For this review, use the dimensioned drawing (mm, ordinates from the lowest corner) and the shaded views. Round coordinates to 2 decimals unless told otherwise and drop trailing zeros. Write each loop counter-clockwise with the first axis right and the second up, starting at its lowest first coordinate (ties: lowest second). Pieces come first, ordered by that corner, then holes.
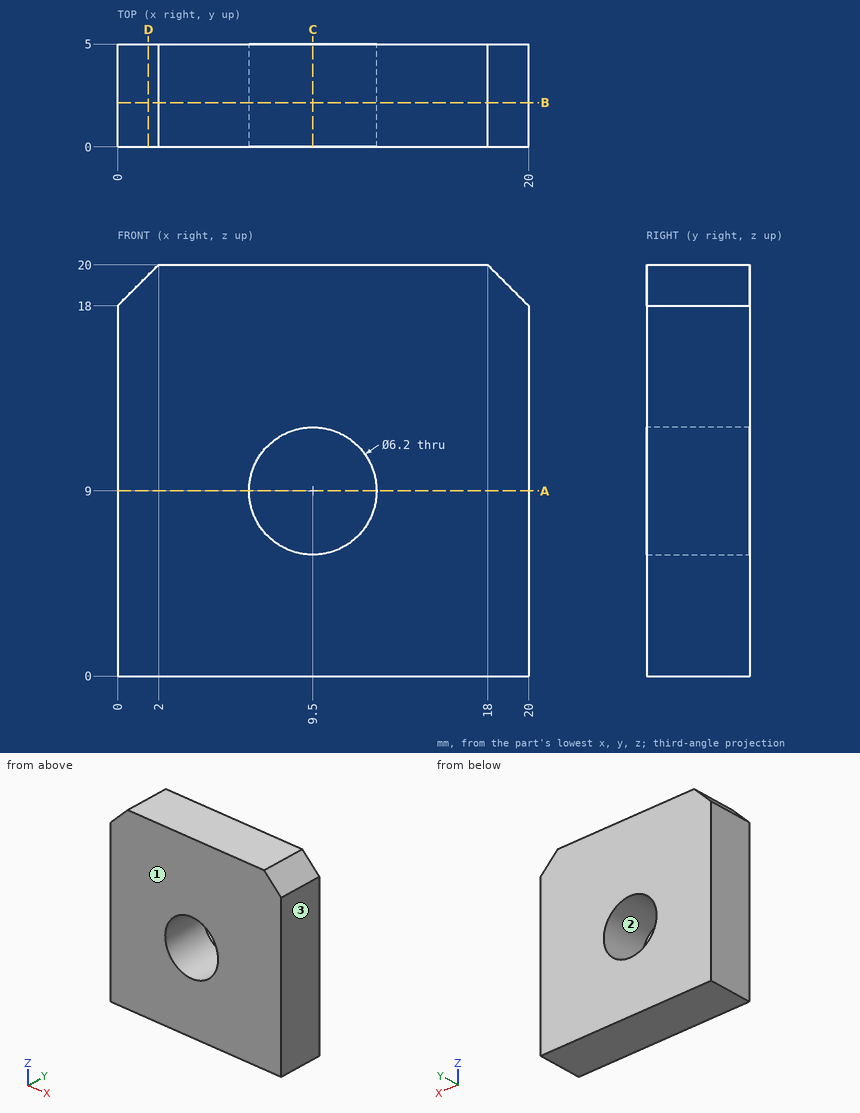
1) Add section C-C on x = 9.5. State the section outline as (y, z) points, and give its area (3 significant figures).
2) Add section B-B on y = 2.15. State the section outline as (x, z) points, and give its area (3 significant figures).
3) Add section D-D on x = 1.5. State the section outline as (y, z) points.
4) For line 1 along X through (y, z) = (2.45, 9); line 2 along Z through (x, y) = (9.75, 2.65); line 3 along X through (y, z) = (4.3, 11), list the stretches that pass through material, from the lowest coordinate up.
5) The part is to be moulded in two halves that separate along X. For the marked faces 1, 2 and 3, say which applies: pulls with the +X half, pulls with the -X half, needs draft (parallel to the pull), parting line crosses it, or undercut.
6) Add section A-A on z = 9. State the section outline as (x, y) points, and give its area (3 significant figures).
Computed:
1. outline: (0, 0) - (5, 0) - (5, 5.9) - (0, 5.9) - close; (0, 12.1) - (5, 12.1) - (5, 20) - (0, 20) - close
1. area: 69.0 mm2
2. outline: (0, 0) - (20, 0) - (20, 18) - (18, 20) - (2, 20) - (0, 18) - close; hole circle Ø6.2 at (9.5, 9)
2. area: 366 mm2
3. outline: (0, 0) - (5, 0) - (5, 19.5) - (0, 19.5) - close
4. line 1: x = 0 to 6.4, 12.6 to 20
4. line 2: z = 0 to 5.91, 12.09 to 20
4. line 3: x = 0 to 7.13, 11.87 to 20
5. face 1: needs draft
5. face 2: undercut
5. face 3: pulls with the +X half
6. outline: (0, 0) - (6.4, 0) - (6.4, 5) - (0, 5) - close; (12.6, 0) - (20, 0) - (20, 5) - (12.6, 5) - close
6. area: 69.0 mm2
